Check sheet for the modelled part. Datum: model origin and axes. Units: mm. A direction names the side the tool comes from. Round coordinates to 2 decimals unless told otherwise and drop trailing zeros. Write each loop counter-clockwise with the first axis right and the second up, starting at its lowest first coordinate (ties: lowest second). Pieces come first, ordered by that corner, then holes. Notation, with made-up numbers: (-32, 58.5) -> (-25, 58.5) arc R13 ccw to (-25, 63.5) -> close; hole circle Ø5 at (75, -6). An arc over 180 degrees is marked (long way). One line per item, written item: value. Start each with the question number.
```python
from build123d import *

# Parameters (mm, degrees)
BOSS_EXTRUDE1_DEPTH = 3
BOSS_EXTRUDE2_DEPTH = 3
BOSS_EXTRUDE4_DEPTH = 3
SKETCH4_R           = 1.4
CUT_EXTRUDE5_DEPTH  = 3
SKETCH5_R           = 2.4
CUT_EXTRUDE6_DEPTH  = 2
SKETCH6_W           = 0.314102564
SKETCH6_H           = 2.557692308
SKETCH6_W_2         = 0.314102565
SKETCH6_H_2         = 3.58974359
CUT_EXTRUDE7_DEPTH  = 1


with BuildPart() as part:
    # Sketch1 → Boss-Extrude1 (new body)
    with BuildSketch(Plane.XY):
        with BuildLine():
            Line((0, 10), (36, 10))
            ThreePointArc((36, 10), (46, 0), (36, -10))
            Line((36, -10), (0, -10))
            ThreePointArc((0, -10), (-10, 0), (0, 10))
        make_face()
    extrude(amount=BOSS_EXTRUDE1_DEPTH)

    # Sketch2 → Boss-Extrude2 (add)
    with BuildSketch(Plane.XY):
        with BuildLine():
            Line((5.104260767, -8.599216361), (-12.094171954, -18.807737895))
            ThreePointArc((-12.094171954, -18.807737895), (-25.797649082, -15.312782302), (-22.302693489, -1.609305174))
            Line((-22.302693489, -1.609305174), (-5.104260767, 8.599216361))
            ThreePointArc((-5.104260767, 8.599216361), (8.599216361, 5.104260767), (5.104260767, -8.599216361))
        make_face()
    extrude(amount=BOSS_EXTRUDE2_DEPTH)

    # Sketch3 → Boss-Extrude4 (add)
    with BuildSketch(Plane.XY):
        with BuildLine():
            Line((-9.998884105, -17.148730445), (-26.65538549, -34.427647124))
            ThreePointArc((-26.65538549, -34.427647124), (-40.795143017, -34.68698683), (-41.054482723, -20.547229303))
            Line((-41.054482723, -20.547229303), (-24.397981338, -3.268312624))
            ThreePointArc((-24.397981338, -3.268312624), (-10.258223811, -3.008972918), (-9.998884105, -17.148730445))
        make_face()
    extrude(amount=BOSS_EXTRUDE4_DEPTH)

    # Sketch4 → Cut-Extrude5 (cut)
    with BuildSketch(Plane.XY):
        with Locations((35.538598823, 0)):
            Circle(SKETCH4_R)
    extrude(amount=CUT_EXTRUDE5_DEPTH, mode=Mode.SUBTRACT)

    # Sketch5 → Cut-Extrude6 (cut)
    with BuildSketch(Plane.XY.offset(3)):
        with Locations((35.538598823, 0)):
            Circle(SKETCH5_R)
    extrude(amount=-CUT_EXTRUDE6_DEPTH, mode=Mode.SUBTRACT)

    # Sketch6 → Cut-Extrude7 (cut)
    # profile 1 of 7: a face of its own
    with BuildSketch(Plane.XY.offset(3)):
        Polygon((9.822398538, 1.128373328), (10.136501102, 1.128373328), (10.136501102, -2.012652313), (11.482654948, -2.012652313), (11.482654948, -2.371626672), (9.822398538, -2.371626672), align=None)
    # profile 2 of 7: a face of its own
    with BuildSketch(Plane.XY.offset(3)):
        with BuildLine():
            add(Edge.make_bspline(
                [(12.087021935, 1.262988713), (12.106513251, 1.26208456), (12.144680991, 1.260314056), (12.199874258, 1.245152579), (12.250131271, 1.219452894), (12.294709003, 1.184973213), (12.33296089, 1.144423769), (12.3597416, 1.097162801), (12.376953997, 1.046104162), (12.379032552, 1.010489073), (12.380090845, 0.9923557)],
                knots=[0, 0, 0, 0, 1.055194115, 2.066272739, 3.074728998, 4.095836921, 5.109056067, 6.073838105, 7.019297344, 8, 8, 8, 8], degree=3))
            add(Edge.make_bspline(
                [(12.380090845, 0.9923557), (12.379008686, 0.974693047), (12.376869384, 0.939776072), (12.359754895, 0.889602599), (12.332732658, 0.842998316), (12.294733532, 0.802527606), (12.250124771, 0.768066986), (12.199875985, 0.742362247), (12.144680537, 0.72720211), (12.106513097, 0.725431421), (12.087021935, 0.724527174)],
                knots=[0, 0, 0, 0, 0.96129708, 1.900370562, 2.859976407, 3.87933698, 4.906634145, 5.921202961, 6.938410037, 8, 8, 8, 8], degree=3))
            add(Edge.make_bspline(
                [(12.087021935, 0.724527174), (12.06775366, 0.725396894), (12.03025048, 0.727089691), (11.975883637, 0.742659709), (11.926055148, 0.768075782), (11.881390475, 0.802301967), (11.844160282, 0.843246864), (11.817061957, 0.889574158), (11.799986995, 0.939783313), (11.797842366, 0.974695479), (11.796757512, 0.9923557)],
                knots=[0, 0, 0, 0, 1.054934014, 2.053291228, 3.073705704, 4.106921865, 5.123545215, 6.088680038, 7.033164197, 8, 8, 8, 8], degree=3))
            add(Edge.make_bspline(
                [(11.796757512, 0.9923557), (11.797818599, 1.010486549), (11.79990264, 1.046096682), (11.817074756, 1.097191715), (11.843934564, 1.144173217), (11.881415127, 1.185198716), (11.926048587, 1.219444151), (11.975885333, 1.244855132), (12.030250032, 1.260426472), (12.067753508, 1.262119086), (12.087021935, 1.262988713)],
                knots=[0, 0, 0, 0, 0.98631895, 1.937192651, 2.907499808, 3.917963147, 4.944918757, 5.95915025, 6.951458133, 8, 8, 8, 8], degree=3))
        make_face()
    # profile 3 of 7: a face of its own
    with BuildSketch(Plane.XY.offset(3)):
        with Locations((12.088424179, -1.092780518)):
            Rectangle(SKETCH6_W, SKETCH6_H)
    # profile 4 of 7: a face of its own
    with BuildSketch(Plane.XY.offset(3)):
        Polygon((13.322398538, 1.218116918), (13.636501102, 1.218116918), (13.636501102, 0.186065636), (14.085219051, 0.186065636), (14.085219051, -0.128036928), (13.636501102, -0.128036928), (13.636501102, -2.371626672), (13.322398538, -2.371626672), (13.322398538, -0.128036928), (12.873680589, -0.128036928), (12.873680589, 0.186065636), (13.322398538, 0.186065636), align=None)
    # profile 5 of 7: a face of its own
    with BuildSketch(Plane.XY.offset(3)):
        Polygon((14.937783153, 1.218116918), (15.251885717, 1.218116918), (15.251885717, 0.186065636), (15.700603666, 0.186065636), (15.700603666, -0.128036928), (15.251885717, -0.128036928), (15.251885717, -2.371626672), (14.937783153, -2.371626672), (14.937783153, -0.128036928), (14.489065204, -0.128036928), (14.489065204, 0.186065636), (14.937783153, 0.186065636), align=None)
    # profile 6 of 7: a face of its own
    with BuildSketch(Plane.XY.offset(3)):
        with Locations((16.351244691, -0.576754877)):
            Rectangle(SKETCH6_W_2, SKETCH6_H_2)
    # profile 7 of 7: a face of its own
    with BuildSketch(Plane.XY.offset(3)):
        with BuildLine():
            Line((19.325403345, -1.563934364), (19.60444982, -1.71046882))
            add(Edge.make_bspline(
                [(19.60444982, -1.71046882), (19.582213225, -1.749912151), (19.538949616, -1.826653254), (19.464548868, -1.932085114), (19.386556796, -2.02693283), (19.301452828, -2.108662484), (19.211783149, -2.179913869), (19.117050494, -2.242251694), (19.016761676, -2.295370214), (18.910911951, -2.340122742), (18.7986124, -2.374532236), (18.679590884, -2.398836457), (18.553619388, -2.413859726), (18.467273209, -2.415604867), (18.423059595, -2.416498467)],
                knots=[0, 0, 0, 0, 1.120438281, 2.179929193, 3.190490725, 4.156257408, 5.095198341, 6.022838206, 6.959905092, 7.901321166, 8.864066838, 9.862729781, 10.905609505, 12, 12, 12, 12], degree=3))
            add(Edge.make_bspline(
                [(18.423059595, -2.416498467), (18.373917618, -2.415351292), (18.278055856, -2.413113485), (18.138516109, -2.39382102), (18.007136691, -2.362348662), (17.883924987, -2.31838312), (17.769182735, -2.260955796), (17.66268188, -2.190996314), (17.563862354, -2.10886406), (17.475838145, -2.013847616), (17.396594262, -1.912165659), (17.326668442, -1.806209774), (17.268211011, -1.69624655), (17.220658401, -1.582976026), (17.182253536, -1.467112132), (17.155486832, -1.347600665), (17.140057084, -1.224765081), (17.137692639, -1.141667745), (17.136501102, -1.099791736)],
                knots=[0, 0, 0, 0, 1.145258523, 2.234067595, 3.276747158, 4.290159414, 5.277019952, 6.260822364, 7.254936242, 8.264827045, 9.274100331, 10.257902744, 11.220704747, 12.172965371, 13.118907548, 14.062713208, 15.023725156, 16, 16, 16, 16], degree=3))
            add(Edge.make_bspline(
                [(17.136501102, -1.099791736), (17.137560243, -1.060496906), (17.139659321, -0.982619741), (17.152890109, -0.867354197), (17.176338402, -0.755325744), (17.208514726, -0.646441296), (17.250065972, -0.540883162), (17.300898191, -0.438587098), (17.361090569, -0.339661959), (17.407563243, -0.277258825), (17.430972256, -0.24582539)],
                knots=[0, 0, 0, 0, 1.024358464, 2.0301432, 3.019427413, 4.004406732, 4.986367066, 5.972626655, 6.978780325, 8, 8, 8, 8], degree=3))
            add(Edge.make_bspline(
                [(17.430972256, -0.24582539), (17.462679938, -0.20795652), (17.525090885, -0.133418369), (17.63064724, -0.035480044), (17.744947437, 0.046563731), (17.866559063, 0.114570868), (17.996895537, 0.166244515), (18.134204828, 0.204752097), (18.280050414, 0.226330108), (18.379755635, 0.229377941), (18.430771935, 0.23093743)],
                knots=[0, 0, 0, 0, 1.030682036, 2.02871468, 2.997146059, 3.962720338, 4.930598197, 5.918074684, 6.934738563, 8, 8, 8, 8], degree=3))
            add(Edge.make_bspline(
                [(18.430771935, 0.23093743), (18.48321954, 0.229583382), (18.586109786, 0.226927046), (18.736141907, 0.202300713), (18.878102624, 0.163248158), (19.011935128, 0.108094368), (19.137652989, 0.036934816), (19.254439039, -0.051207025), (19.364290551, -0.153625113), (19.42819913, -0.232388322), (19.460719852, -0.272468018)],
                knots=[0, 0, 0, 0, 1.056321875, 2.072262726, 3.055038591, 4.01806755, 4.982017516, 5.957941055, 6.960871419, 8, 8, 8, 8], degree=3))
            add(Edge.make_bspline(
                [(19.460719852, -0.272468018), (19.48284679, -0.3026716), (19.526953383, -0.362877718), (19.582200483, -0.461048875), (19.630157878, -0.56375947), (19.668490839, -0.672669767), (19.69953034, -0.786489347), (19.721987159, -0.906031892), (19.735156778, -1.031261803), (19.737745475, -1.116588359), (19.739065204, -1.160088211)],
                knots=[0, 0, 0, 0, 0.94817472, 1.890038105, 2.849395472, 3.817997239, 4.812318967, 5.836947057, 6.897266129, 8, 8, 8, 8], degree=3))
            Line((19.739065204, -1.160088211), (17.450603666, -1.160088211))
            add(Edge.make_bspline(
                [(17.450603666, -1.160088211), (17.452143272, -1.193788675), (17.455170846, -1.260059279), (17.469285989, -1.357030062), (17.491534763, -1.449403404), (17.522803826, -1.536486446), (17.560670671, -1.619416573), (17.607056388, -1.69757861), (17.662395942, -1.77061654), (17.724121641, -1.839183678), (17.792828737, -1.900244439), (17.865111484, -1.954896215), (17.942005049, -2.000701812), (18.022903132, -2.037881702), (18.107674917, -2.066988018), (18.196347113, -2.086855839), (18.288745229, -2.100162945), (18.351730963, -2.101642611), (18.383796775, -2.102395903)],
                knots=[0, 0, 0, 0, 1.094153842, 2.151609401, 3.174256925, 4.172055639, 5.149267565, 6.128595816, 7.11444997, 8.118368179, 9.117203808, 10.09244225, 11.054858984, 12.015122123, 12.976791628, 13.957293641, 14.960065497, 16, 16, 16, 16], degree=3))
            add(Edge.make_bspline(
                [(18.383796775, -2.102395903), (18.415147922, -2.101787846), (18.477354613, -2.100581345), (18.569995471, -2.088849434), (18.661134998, -2.069879159), (18.750395981, -2.043989169), (18.835966827, -2.012412316), (18.915212377, -1.974309459), (18.988092593, -1.932159712), (19.05620956, -1.883950037), (19.122280553, -1.82494185), (19.187823039, -1.751306129), (19.258099693, -1.664218601), (19.302089285, -1.598672935), (19.325403345, -1.563934364)],
                knots=[0, 0, 0, 0, 0.99110716, 1.966546729, 2.947904876, 3.932708344, 4.903319531, 5.828989031, 6.710028674, 7.56322171, 8.463672341, 9.504779593, 10.677557249, 12, 12, 12, 12], degree=3))
        make_face()
        with BuildLine():
            add(Edge.make_bspline(
                [(19.42496264, -0.845985646), (19.413466016, -0.804322773), (19.391338714, -0.724135152), (19.34510235, -0.613094262), (19.293030809, -0.514406361), (19.231409078, -0.428826728), (19.161590352, -0.352823215), (19.080945169, -0.286404629), (18.990509276, -0.226987178), (18.890750135, -0.176834679), (18.78510835, -0.13414482), (18.674502158, -0.105519704), (18.56164437, -0.085910162), (18.485310084, -0.084084054), (18.446897736, -0.083165134)],
                knots=[0, 0, 0, 0, 1.154881502, 2.222775134, 3.210006277, 4.132804581, 5.035138423, 5.962687519, 6.919655026, 7.923214229, 8.944639381, 9.960483929, 10.97369054, 12, 12, 12, 12], degree=3))
            add(Edge.make_bspline(
                [(18.446897736, -0.083165134), (18.415548298, -0.083776805), (18.353577049, -0.084985951), (18.262275981, -0.096456081), (18.174596282, -0.115415925), (18.089890994, -0.141380882), (18.009270126, -0.175989485), (17.931075358, -0.216572711), (17.857294961, -0.266114295), (17.811153666, -0.30387315), (17.787843249, -0.322948787)],
                knots=[0, 0, 0, 0, 1.04873581, 2.073130211, 3.073294108, 4.04793562, 5.032784715, 6.005352987, 6.992311501, 8, 8, 8, 8], degree=3))
            add(Edge.make_bspline(
                [(17.787843249, -0.322948787), (17.771149967, -0.338043103), (17.737366833, -0.368590319), (17.692226312, -0.421219526), (17.649005839, -0.477971088), (17.609672186, -0.541016212), (17.5735946, -0.609636991), (17.539834622, -0.683254627), (17.50944821, -0.762427757), (17.4923521, -0.817600196), (17.48355639, -0.845985646)],
                knots=[0, 0, 0, 0, 0.879870761, 1.780643979, 2.707998968, 3.669668524, 4.684282772, 5.740141944, 6.837334558, 8, 8, 8, 8], degree=3))
            Line((17.48355639, -0.845985646), (19.42496264, -0.845985646))
        make_face(mode=Mode.SUBTRACT)
    extrude(amount=-CUT_EXTRUDE7_DEPTH, mode=Mode.SUBTRACT)


solid = part.part
```
1. Cross-section at B-B (y = -7). Record the cut outline in (x, z).
2. Access from +Z, -Z, +X, -X, +Y, -Y to the whole of each face (thin tool, end or side, straight path). Record for faces 5 (the face through (33.14, 0.11, 2.01)), 6 (the face through (-18.685, -26.159, 1.479)).
3. Depth check by flat-ended pin: pin 1 Ø0.8 at (y, z) = (-0.5, 2.5) entering from -X; pin 2 Ø0.5 at (y, z) = (-1.5, 2.5) entering from +X; pin 3 Ø1.5 at (x, z) = (27.5, 0.5) entering from -Y. Enter the tip coordinate at first touch or a pass-through.
4. Cross-section at C-C (y = 7.5). Record the cut outline in (x, z).
5. Material ranges on probe 1 along Y at (x, z) = (23, 2.45); probe 2 along X at (y, z) = (0.5, 1.5); probe 3 along X at (y, z) = (-23.5, 2.35), recorded low to high.
6. Cross-section at A-A (x = 35). Record the cut outline in (y, z).
7. Release check for a two-part mould opening along Y. For faces 1 (the face through (9.98, -1, 2)), 2 (the face through (18, -1, 2)), 3 (the face through (20, -10, 1)), 4 (the face through (-40.635, -34.838, 1.479)) record: +Y half, -Y half, draft (parallel to the pull), parting line (faces both ways), or undercut.
Working result:
1. outline: (-28, 0) -> (43.14, 0) -> (43.14, 3) -> (-28, 3) -> close
2. face 5: +Z
2. face 6: +Z, -Z, +X, -Y
3. pin 1: stops at x = -21.11
3. pin 2: stops at x = 45.92
3. pin 3: stops at y = -10
4. outline: (-6.96, 0) -> (42.61, 0) -> (42.61, 3) -> (-6.96, 3) -> close
5. probe 1: y = -10 to 10
5. probe 2: x = -18.75 to 33.19, 37.89 to 45.99
5. probe 3: x = -43.03 to -16.12
6. outline: (-10, 0) -> (-1.29, 0) -> (-1.29, 1) -> (-2.34, 1) -> (-2.34, 3) -> (-10, 3) -> close; (1.29, 0) -> (10, 0) -> (10, 3) -> (2.34, 3) -> (2.34, 1) -> (1.29, 1) -> close
7. face 1: undercut
7. face 2: undercut
7. face 3: -Y half
7. face 4: parting line
